Model file for the job. Use its own axes, mm. Round coordinates to 2 decimals unless told otherwise and drop trailing zeros. Loops run counter-clockwise (first coordinate to the right, second up) from the corner with the lowest first, then second, coordinate; pieces in that order, holes last. Notation, with made-up numbers: M 73.25,44.25 L 85.25,44.25 A22 cw 85.25,54.25 Z; hole C -3,58.25 d9. An arc over 180 degrees is marked long. Answer in a Markdown table with one row per item.
from build123d import *

# Parameters (mm, degrees)
F2_R = 0.5


with BuildPart() as f1:
    # F0 (on Front) → F1 (revolve)
    with BuildSketch(Plane.XZ):
        Polygon((10, 10.5), (2.5, 3), (2.5, 0), (12.5, 0), (12.5, 10.5), align=None)
    revolve(axis=Axis((0, 0, 15.3351295739), (0, 0, -1)))

    # F2
    f2_edges = [f1.edges().sort_by_distance(p)[0] for p in [
        (-12.5, 0, 10.5),
        (-10, 0, 10.5),
        (-2.5, 0, 3),
        (-2.5, 0, 0),
    ]]
    fillet(f2_edges, radius=F2_R)


solid = f1.part
1. Pin check, flat tips, straight feed: pin 1 (5 mm diameter, centred on x = 10, z = 7, fed in from +Y); pin 2 (3 mm diameter, centred on x = -8, z = 3, fed in from +Y); pin 3 (6 mm diameter, centred on x = -5.5, z = 8, fed in from -Y). Stop position of each tip, or through.
Verdict:
| item | result |
|---|---|
| pin 1 | stops at y = 10 |
| pin 2 | stops at y = 10.68 |
| pin 3 | stops at y = -12.25 |
2. Mould opens along X. For faces 1 (the cylindrical face through (11.923, -3.755, 5.07)), 2 (the cylindrical face through (2.385, -0.751, 1.63)), 3 (the flat face through (3, -10, 10.5)) say: +X half, -X half, draft (parallel to the pull), parting line (faces both ways), or undercut.
Verdict:
| item | result |
|---|---|
| face 1 | parting line |
| face 2 | undercut |
| face 3 | draft |
3. Saw through at B-B (z = 9.5). Write the cut outline in (x, y), and give its area (3 significant figures).
Verdict:
| item | result |
|---|---|
| outline | C 0,0 d25; hole C 0,0 d18 |
| area | 236 mm² |
4. Wall check: probe 1 along X at (y, z) = (0, 2.25); probe 2 along X at (y, z) = (-2.25, 8). Give the ranges that are in metal, low to high.
Verdict:
| item | result |
|---|---|
| probe 1 | x = -12.5 to -2.5, 2.5 to 12.5 |
| probe 2 | x = -12.3 to -7.15, 7.15 to 12.3 |
5. Saw through at A-A (z = 5). Write the cut outline in (x, y).
Verdict:
| item | result |
|---|---|
| outline | C 0,0 d25; hole C 0,0 d9 |
